Autodesk Inventor part; units mm, degrees
ref_plane "РабПлоскость1" through (0, -5, 0) normal (0, 0, -1) x (0, 1, 0)
ref_plane "РабПлоскость2" through (0, -5, 45) normal (0, 0, -1) x (0, 1, 0)
ref_plane "YZ Plane" through (0, 0, 0) normal (1, 0, 0) x (0, 1, 0)
sketch "Эскиз1" plane through (0, 0, 0) normal (1, 0, 0) x (0, 1, 0)
  line L0 (0, 0) -> (10, 0)
  line L1 (10, 0) -> (10, 45)
  line L2 (10, 45) -> (0, 45)
  line L3 (0, 45) -> (0, 0)
  arc A0 (10, 45) -> (0, 45) centre (5, 45) ccw
  arc A1 (0, 0) -> (10, 0) centre (5, 0) ccw
  circle A2 centre (5, 45) radius 7.5
  circle A3 centre (5, 0) radius 7.5
  line L4 (0, 22.5) -> (10, 22.5)
  line L5 (0, 27.5) -> (-20, 27.5)
  line L6 (-20, 27.5) -> (-20, 17.5)
  line L7 (-20, 17.5) -> (0, 17.5)
  line L8 (0, 17.5) -> (0, 27.5)
  line L9 (7, 27.5) -> (3, 27.5)
  line L10 (3, 27.5) -> (3, 17.5)
  line L11 (3, 17.5) -> (7, 17.5)
  line L12 (7, 17.5) -> (7, 27.5)
  circle A4 centre (5, 45) radius 10
  circle A5 centre (5, 0) radius 10
  point P0 (0, 17.5)
  point P1 (0, 8.6603)
  point P2 (10, 8.6603)
  point P3 (10, 5.5902)
  point P4 (0, 5.5902)
  point P5 (10, 36.3397)
  point P6 (0, 36.3397)
  point P7 (0, 39.4098)
  point P8 (10, 39.4098)
  dimension "d0" = 45
  dimension "d1" = 10
  dimension "d2" = 15
  dimension "d3" = 15
  dimension "d6" = 10
  dimension "d7" = 20
  dimension "d8" = 10
  dimension "d9" = 20
  dimension "d10" = 20
extrude "Выдавливание1" add sketch "Эскиз1" along normal blind 4 contours A3 L1 A5 L3 | L3 A5 L1 A3 | L3 L4 L10 L11 L12 L1 A5 | L4 L12 L9 L10 L3 A4 L1 | A4 L3 A2 L1 | L1 A2 L3 A4
sketch "Эскиз3" plane through (0, 0, 0) normal (-1, 0, 0) x (0, 0, 1)
  arc A0 (8.6603, 10) -> (8.6603, 0) centre (0, 5) ccw
  line L0 (0, -5) -> (0, 15)
  arc A1 (36.3397, 0) -> (36.3397, 10) centre (45, 5) ccw
  line L1 (45, -5) -> (45, 15)
  point P0 (0, 0)
ref_plane "РабПлоскость1" through (0, -5, 0) normal (0, 0, -1) x (0, 1, 0)
ref_plane "РабПлоскость2" through (0, -5, 45) normal (0, 0, -1) x (0, 1, 0)
sketch "Эскиз4" plane through (0, -5, 0) normal (0, 0, -1) x (0, 1, 0)
  line L0 (20, 0) -> (0, 0)
  line L1 (10, 0) -> (10, -15)
  line L2 (10, -15) -> (20, 0)
  point P0 (5, 0)
  point P1 (15, 0)
  dimension "d15" = 15
revolve "Вращение1" add sketch "Эскиз4" angle 360 about axis through (0, 5, 0) along (-1, 0, 0)
sketch "Эскиз5" plane through (0, -5, 45) normal (0, 0, -1) x (0, 1, 0)
  line L0 (20, 0) -> (10, -15)
  line L1 (20, 0) -> (10, -15)
  line L2 (15, 0) -> (5, 0)
  line L3 (10, 0) -> (10, -15)
  line L4 (20, 0) -> (0, 0)
  line L5 (10, 0) -> (20, 0)
revolve "Вращение2" add sketch "Эскиз5" angle 360 about axis through (0, 5, 45) along (-1, 0, 0)
sketch "Эскиз6" plane through (0, 5, 0) normal (1, 0, 0) x (0, 0, -1)
  arc A0 (-8.6603, -5) -> (-8.6603, 5) centre (0, 0) ccw
  circle A1 centre (0, 0) radius 6.5
  circle A2 centre (-45, 0) radius 7.5
  circle A3 centre (-45, 0) radius 6.5
  point P0 (0, -5)
  dimension "d18" = 13
  dimension "d19" = 13
extrude "Выдавливание3" cut sketch "Эскиз6" against normal blind 2 contours A1 | A3
properties part number "соединение пушек перед"
Here's how the part is built. I have some questions about the finished solid (model axes, mm). A direction names the side the tool comes from. Coordinates: 2 decimals unless noted, no trailing zeros. Order: outer loops, then holes, each group sorted by start corner. A loop starts at its lowest first (then second) coordinate and runs counter-clockwise, first axis right, second up.
Item 1: If we section it at A-A on z = 25.5: List the corners of the cut face in (x, y) for me.
Result sheet:
outline: (0, 0) - (4, 0) - (4, 3) - (0, 3) - close; (0, 7) - (4, 7) - (4, 10) - (0, 10) - close
Item 2: I need wall thicknesses on line 1 (Z direction, x = 1.6, y = 5); line 2 (Z direction, x = -3, y = 2.25); line 3 (Y direction, x = 0.75, z = 24.5). Which ranges of each line are inside material? Lowest first, please.
Result sheet:
line 1: z = -10 to -7.5, 7.5 to 17.5, 27.5 to 37.5, 52.5 to 55
line 2: z = -7.51 to 7.51, 37.49 to 52.51
line 3: y = 0 to 3, 7 to 10
Item 3: If we section it at B-B on x = -12: List the corners of the cut face in (y, z) for me.
Result sheet:
outline: circle Ø4 at (5, 0); circle Ø4 at (5, 45)
Item 4: For P1, Ø5, axis at x = -6.5, y = 12.5, coming from the -Z side; P2, Ø2, axis at x = 1.5, z = 23.5, coming from the +Y side; P3, Ø3, axis at x = 2.5, z = 17, coming from the -Y side, each with a flat end and sliding along its axis, tell me the tip position at first contact or that it passes through.
Result sheet:
P1: stops at z = -3.77
P2: stops at y = 10
P3: stops at y = 0
Item 5: If we mould it in two halves opening along Z, with no side actions, what happens to faces 1 (the face through (-2, 5, 0)), 2 (the face through (-0.986, 1.045, 5.158)), 3 (the face through (4, 2.6, 23))? For each: +Z half, -Z half, draft (parallel to the pull), parting line (faces both ways), or undercut.
Result sheet:
face 1: undercut
face 2: undercut
face 3: draft
Item 6: For faces 4 (the face through (2, 0, 23)), 5 (the face through (2, 5, 27.5)), 6 (the face through (1.97, 11.93, 2.87)), 7 (the face through (2, 10, 22)), which set-ups out of +Z, -Z, +X, -X, +Y, -Y let a thin tool reach every point of the face, with its end or its side?
Result sheet:
face 4: +X, -X, -Y
face 5: +X, -X
face 6: +X
face 7: +X, -X, +Y
Item 7: If we section it at C-C on x = -6: List the corners of the cut face in (y, z) for me, plus the area to 3 significant figures.
Result sheet:
outline: circle Ø12 at (5, 0); circle Ø12 at (5, 45)
area: 226 mm2
